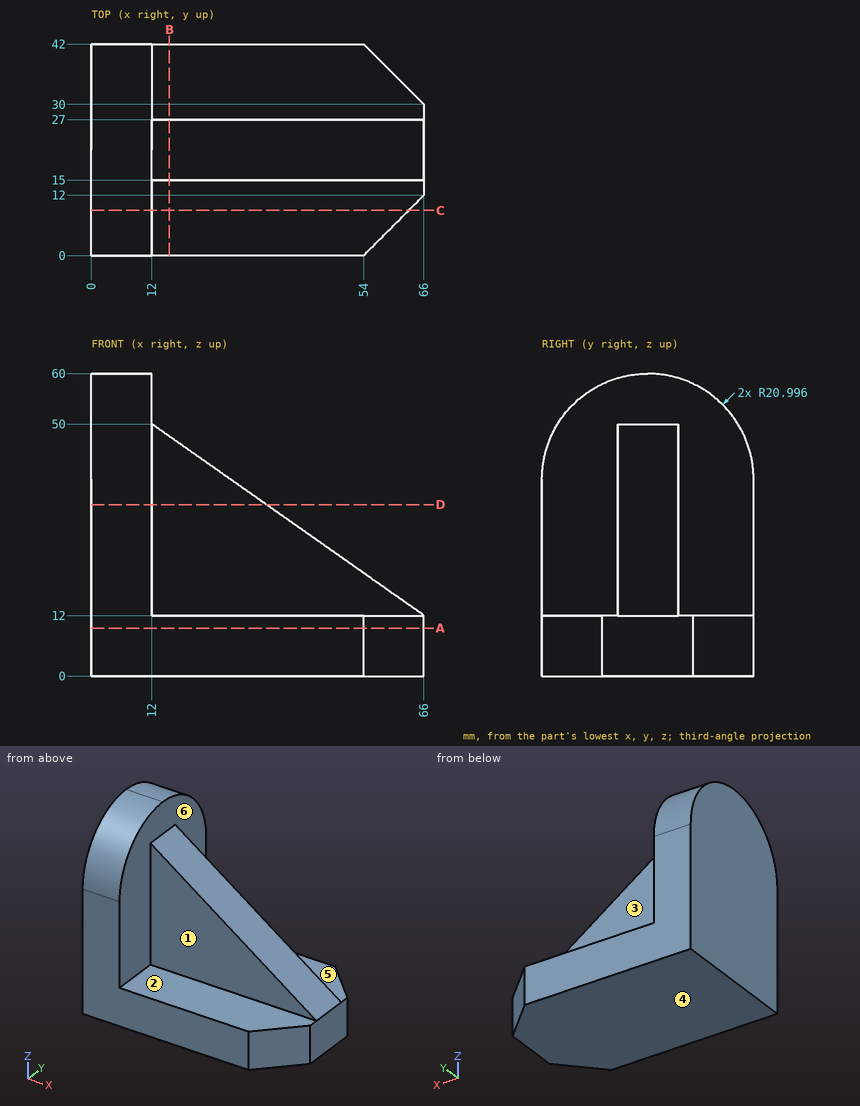
Answer from the drawing. Dimensions are ordinates in mm from the lowest x, y and z of the part. A direction names the side the tool comes from. Coordinates: 2 decimals unless noted, no trailing zeros. Write each loop counter-clockwise with the first axis right and the second up, starting at its lowest first coordinate (ties: lowest second). Pieces come first, ordered by that corner, then holes. Notation, with made-up numbers: M 24.25,39.5 L 42.25,39.5 A12 ccw 42.25,53.5 Z; hole C -35,70.5 d11. An arc over 180 degrees is marked long. Use one line per item in the form item = value. Start each with the question number.
1. The part is cut by section B-B (x = 15.5). Give the vertices of the cut face in (y, z).
2. The mould has two halves that part along Y. Classify the marked faces 1, 2 and 3: released by +Y, released by -Y, zero draft, split by the parting line, or undercut.
3. Straight lines are drawn through the part: probe 1 along Z at (x, y) = (55, 28); probe 2 along Y at (x, z) = (52, 18). For each, find the intervals that lie inside material, in ascending order. Write a range as from..to.
4. The part is cut by section A-A (z = 9.5). Give the vertices of the cut face in (x, y).
5. The part is cut by section D-D (z = 34). Give the vertices of the cut face in (x, y), plus the area to 3 significant figures.
6. Each of these flat-tipped pins is pushed along its axis until it touches: P1, Ø4, axis at y = 15.5, z = 42, coming from the +X side; P2, Ø4.5, axis at x = 42, y = 8, coming from the +Z side; P3, Ø19, axis at x = 37, z = 30, coming from the -Y side. Where does it stop, or does it pass through?
7. A tool of negligible diameter and unlimited length cuts with its end or side. For the marked faces 4, 5 and 6, from which of +Z, -Z, +X, -X, +Y, -Y can it reach the whole face along a straight path? Write none if from no direction.
8. The part is cut by section C-C (y = 9). Give the vertices of the cut face in (x, z), plus the area to 3 significant figures.
Evaluation:
q1.outline = M 0,0 L 42,0 L 42,12 L 27,12 L 27,47.54 L 15,47.54 L 15,12 L 0,12 Z
q2.face_1 = released by -Y
q2.face_2 = zero draft
q2.face_3 = released by +Y
q3.probe_1 = 0..12
q3.probe_2 = 15..27
q4.outline = M 0,0 L 54,0 L 66,12 L 66,30 L 54,42 L 0,42 Z
q5.outline = M 0,0 L 12,0 L 12,15 L 34.74,15 L 34.74,27 L 12,27 L 12,42 L 0,42 Z
q5.area = 777 mm^2
q6.P1 = 26.21
q6.P2 = 12
q6.P3 = 15
q7.face_4 = -Z, +X, -X, +Y, -Y
q7.face_5 = +Z, +X, +Y
q7.face_6 = +Z, +X
q8.outline = M 0,0 L 63,0 L 63,12 L 12,12 L 12,56.24 L 0,56.24 Z
q8.area = 1,290 mm^2
